The model under review builds one solid part; all positions refer to its coordinate system, in mm. A direction names the side the tool comes from. Round coordinates to 2 decimals unless told otherwise and drop trailing zeros. Order: outer loops, then holes, each group sorted by start corner. A loop starts at its lowest first (then second) coordinate and runs counter-clockwise, first axis right, second up. Notation, with made-up numbers: M 35,-34 L 91,-34 A35 ccw 91,2 Z; hole C -17,-38 d10. An arc over 180 degrees is marked long. One line per item, written item: value. Start each with the question number.
Autodesk Inventor part; units mm, degrees
ref_plane "YZ Plane" through (0, 0, 0) normal (1, 0, 0) x (0, 1, 0)
ref_plane "XZ Plane" through (0, 0, 0) normal (0, 1, 0) x (-1, 0, 0)
ref_plane "XY Plane" through (0, 0, 0) normal (0, 0, 1) x (1, 0, 0)
sketch "Sketch1" plane through (0, 0, 0) normal (1, 0, 0) x (0, 1, 0)
  line L0 (25.4, 25.4) -> (-25.4, 25.4)
  line L1 (-25.4, 25.4) -> (-25.4, -25.4)
  line L2 (-25.4, -25.4) -> (25.4, -25.4)
  line L3 (25.4, -25.4) -> (25.4, 25.4)
  line L4 (23.2918, 23.2918) -> (-23.2918, 23.2918)
  line L5 (-23.2918, 23.2918) -> (-23.2918, -23.2918)
  line L6 (-23.2918, -23.2918) -> (23.2918, -23.2918)
  line L7 (23.2918, -23.2918) -> (23.2918, 23.2918)
  point P0 (0, 0)
  point P1 (0, -25.4)
  point P2 (25.4, 0)
  dimension "d0" = 50.8
  dimension "d1" = 50.8
  dimension "d2" = 2.1082
extrude "Extrusion1" add sketch "Sketch1" along normal blind 1524
fillet "Fillet1" radius 3.175 4 edges at (762, 25.4, 25.4) (762, -25.4, 25.4) (762, 25.4, -25.4) (762, -25.4, -25.4)
properties part number "60_inch_square" material "Steel"
Item 1: Consider section A-A, the plane y = -4.5. Give the boundary of the cut face in (x, z).
Item 2: Consider section C-C, the plane x = 336. Give the boundary of the cut face in (y, z) (3 decimals), then the cut area to 3 significant figures.
Item 3: Wall thickness on L1, parallel to Z at x = 783, y = 8; L2, parallel to Z at x = 869, y = -23: over which ranges is each line inside the solid? List them lowest first.
Item 4: Machinability: for faces 1 (the flat face through (0, 0, -24)), 2 (the flat face through (751, 0, 23.292)), which of the approach directions +Z, -Z, +X, -X, +Y, -Y give a long, thin tool a straight path to every point of the face, cutting with its end or side? Answer none if there is none.
Computed:
1. outline: M 0,-25.4 L 1524,-25.4 L 1524,-23.29 L 0,-23.29 Z; M 0,23.29 L 1524,23.29 L 1524,25.4 L 0,25.4 Z
2. outline: M -25.4,-22.225 A3.175 ccw -22.225,-25.4 L 22.225,-25.4 A3.175 ccw 25.4,-22.225 L 25.4,22.225 A3.175 ccw 22.225,25.4 L -22.225,25.4 A3.175 ccw -25.4,22.225 Z; hole M -23.292,-23.292 L 23.292,-23.292 L 23.292,23.292 L -23.292,23.292 Z
2. area: 402 mm^2
3. L1: z = -25.4 to -23.29, 23.29 to 25.4
3. L2: z = -25.3 to -23.29, 23.29 to 25.3
4. face 1: +Z, -Z, -X, +Y, -Y
4. face 2: +X, -X
